Here's how the part is built. I have some questions about the finished solid (model axes, mm). A direction names the side the tool comes from. Coordinates: 2 decimals unless noted, no trailing zeros. Write each loop counter-clockwise with the first axis right and the second up, starting at its lowest first coordinate (ties: lowest second). Pieces come first, ordered by that corner, then holes.
Item 1: I want a section at B-B (x = 0). Please give me the cut outline in (y, z), and give its area (3 significant figures).
Item 2: I'm going to push flat-ended pins straight in: P1, Ø11.5, axis at x = 0, z = 0, coming from the -Y side; P2, Ø6, axis at x = -3, y = 40, coming from the -Z side; P3, Ø3, axis at y = 27, z = -0.5, coming from the -X side; P4, Ø4, axis at y = 41, z = -13.5, coming from the +X side. Where does each tip first touch, or does it pass through?
Item 3: Please list where these lines run through material, in increasing order: line 1 (Z direction, x = 0, y = 11); line 2 (X direction, y = 18, z = 1); line 3 (Y direction, x = -9, z = -13).
Item 4: If we mould it in two halves opening along X, with no side actions, what happens to faces 3 (the face through (-1.08, 25.42, -4.88)), 4 (the face through (-4, -5, 5)), 5 (the face through (0, -2, 20))? For each: pulls with the +X half, pulls with the -X half, needs draft (parallel to the pull), parting line crosses it, or undercut.
Item 5: For faces 1 (the face through (-4, 0, 15)), 2 (the face through (16, -2, 0)), which set-ups out of +Z, -Z, +X, -X, +Y, -Y let a thin tool reach every point of the face, with its end or its side?
Item 6: I want a section at D-D (y = 43.5). Please give me the cut outline in (x, z), and give its area (3 significant figures).
Item 7: I want a section at C-C (y = 33). Please give me the cut outline in (x, z).
Item 8: I want a section at A-A (z = 0). Please give me the cut outline in (x, y), and give its area (3 significant figures).
from build123d import *

# Parameters (mm, degrees)
F1_DEPTH = 5
F2_R     = 15
F3_DEPTH = 55
F4_R     = 5
F5_DEPTH = 55
F6_DEPTH = 5


with BuildPart() as f1:
    # F0 (on Front) → F1 (new body)
    with BuildSketch(Plane.XZ):
        with BuildLine():
            Line((16, 0), (16, 12))
            ThreePointArc((16, 12), (0, 20), (-16, 12))
            Line((-16, 12), (-16, 0))
            Line((-16, 0), (0, 0))
            Line((0, 0), (16, 0))
        make_face()
        with BuildLine():
            ThreePointArc((-16, -12), (0, -20), (16, -12))
            Line((16, -12), (16, 0))
            Line((16, 0), (0, 0))
            Line((0, 0), (-16, 0))
            Line((-16, 0), (-16, -12))
        make_face()
    extrude(amount=F1_DEPTH)

    # F2 (on face) → F3 (join)
    with BuildSketch(Plane.XZ):
        Circle(F2_R)
    extrude(amount=-F3_DEPTH)

    # F4 (on Front) → F5 (cut, through all)
    with BuildSketch(Plane.XZ):
        Circle(F4_R)
    extrude(amount=-F5_DEPTH, mode=Mode.SUBTRACT)

    # F4 (on Front) → F6 (cut, through all)
    with BuildSketch(Plane.XZ):
        Circle(F4_R)
    extrude(amount=F6_DEPTH, mode=Mode.SUBTRACT)

    # F7 (on Right) → F8 (revolve, cut)
    with BuildSketch(Plane.YZ):
        with BuildLine():
            Line((45, 15), (42.5, 15))
            ThreePointArc((42.5, 15), (45, 12.5), (47.5, 15))
            Line((47.5, 15), (45, 15))
        make_face()
    revolve(axis=Axis((0, 0, 0), (0, -1, 0)), mode=Mode.SUBTRACT)

    # F7 (on Right) → F9 (revolve, cut)
    with BuildSketch(Plane.YZ):
        Polygon((54, 15), (55, 14), (55, 15), align=None)
    revolve(axis=Axis((0, 0, 0), (0, -1, 0)), mode=Mode.SUBTRACT)


solid = f1.part
Answer:
1. outline: (-5, -20) - (0, -20) - (0, -15) - (42.5, -15) arc R2.5 cw to (47.5, -15) - (54, -15) - (55, -14) - (55, -5) - (-5, -5) - close; (-5, 5) - (55, 5) - (55, 14) - (54, 15) - (47.5, 15) arc R2.5 cw to (42.5, 15) - (0, 15) - (0, 20) - (-5, 20) - close
1. area: 1,230 mm2
2. P1: stops at y = -5
2. P2: stops at z = -15
2. P3: stops at x = -15
2. P4: stops at x = 9.63
3. line 1: z = -15 to -5, 5 to 15
3. line 2: x = -14.97 to -4.9, 4.9 to 14.97
3. line 3: y = -5 to 0
4. face 3: undercut
4. face 4: needs draft
4. face 5: parting line crosses it
5. face 1: +Y
5. face 2: +Z, -Z, +X, +Y, -Y
6. outline: circle Ø26 at (0, 0); hole circle Ø10 at (0, 0)
6. area: 452 mm2
7. outline: circle Ø30 at (0, 0); hole circle Ø10 at (0, 0)
8. outline: (-16, -5) - (-5, -5) - (-5, 55) - (-14, 55) - (-15, 54) - (-15, 47.5) arc R2.5 cw to (-15, 42.5) - (-15, 0) - (-16, 0) - close; (5, -5) - (16, -5) - (16, 0) - (15, 0) - (15, 42.5) arc R2.5 cw to (15, 47.5) - (15, 54) - (14, 55) - (5, 55) - close
8. area: 1,190 mm2
